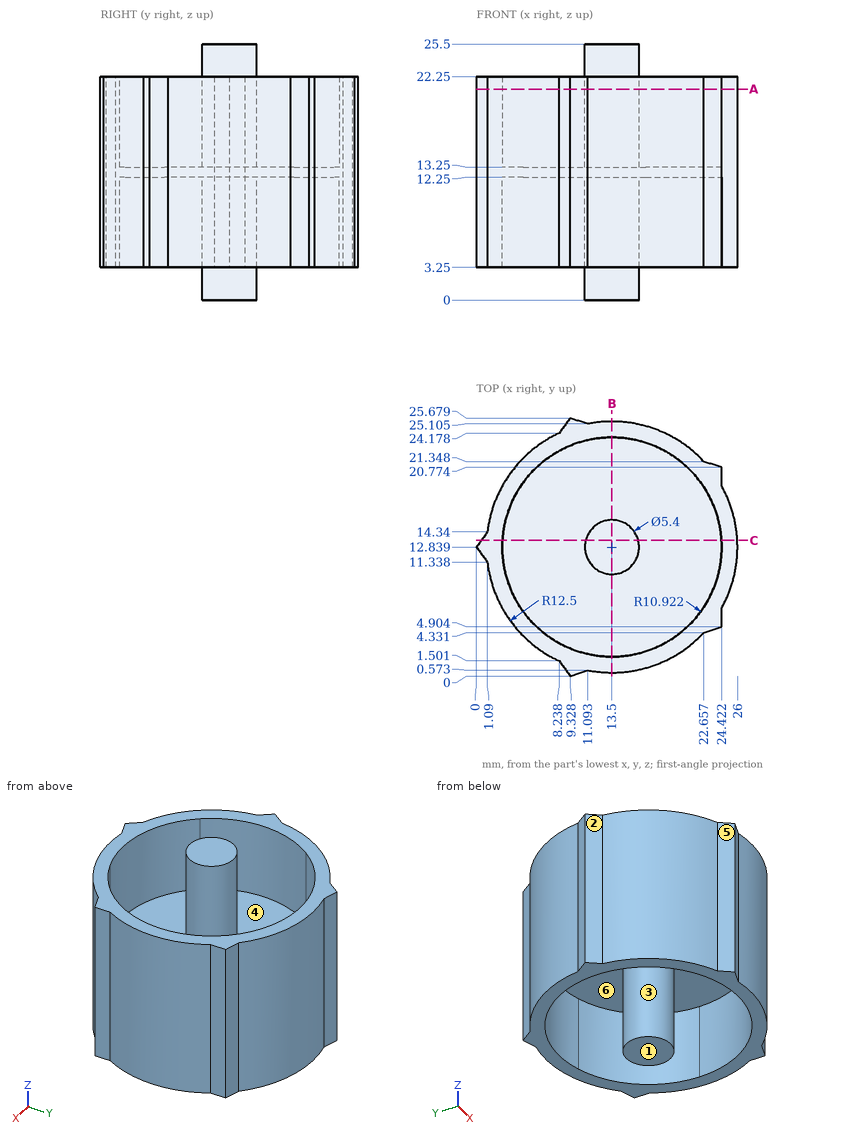
Here's the drawing with two shaded views (mm, measured from the low corner). I have some questions. A direction names the side the tool comes from. Round coordinates to 2 decimals unless told otherwise and drop trailing zeros. Write each loop counter-clockwise with the first axis right and the second up, starting at its lowest first coordinate (ties: lowest second). Pieces come first, ordered by that corner, then holes. Notation, with made-up numbers: M 6,-30.75 L 20,-30.75 A33 cw 20,-2.75 Z; hole C 36.25,43 d3. An arc over 180 degrees is marked long. Use CSV: the item, a comma, the result in double quotes.
(1) We'd pull the mould along X, two halves only. Please class the marked faces 1, 2 and 3: +X half, -X half, draft (parallel to the pull), parting line (faces both ways), or undercut.
Check values:
face 1,"draft"
face 2,"-X half"
face 3,"undercut"
(2) I need wall thicknesses on line 1 along X through (y, z) = (12, 7.75) (1 decimal); line 2 along Z through (x, y) = (8.25, 7.75); line 3 along Y through (x, z) = (22, 21.75) (1 decimal). Which ranges of each line are inside material? Lowest first, please.
Check values:
line 1,"0.6 to 2.6, 10.9 to 16.1, 24.4 to 26"
line 2,"12.25 to 13.25"
line 3,"3.7 to 6, 19.7 to 22"
(3) Imagine slicing it at B-B (x = 13.5). Write out the boundary of the cut face in (y, z).
Check values:
outline,"M 0.34,3.25 L 1.92,3.25 L 1.92,12.25 L 10.14,12.25 L 10.14,0 L 15.54,0 L 15.54,12.25 L 23.76,12.25 L 23.76,3.25 L 25.34,3.25 L 25.34,22.25 L 23.76,22.25 L 23.76,13.25 L 15.54,13.25 L 15.54,25.5 L 10.14,25.5 L 10.14,13.25 L 1.92,13.25 L 1.92,22.25 L 0.34,22.25 Z"
(4) Imagine slicing it at A-A (z = 21). Write out the boundary of the cut face in (x, y) (1 decimal), plus the area to 3 significant figures.
Check values:
outline,"M 0,12.8 L 1.1,11.3 A12.5 ccw 8.2,1.5 L 9.3,0 L 11.1,0.6 A12.5 ccw 22.7,4.3 L 24.4,4.9 L 24.4,6.8 A12.5 ccw 24.4,18.9 L 24.4,20.8 L 22.7,21.3 A12.5 ccw 11.1,25.1 L 9.3,25.7 L 8.2,24.2 A12.5 ccw 1.1,14.3 Z; C 13.5,12.8 d5.4; hole C 13.5,12.8 d21.8"
area,"146 mm^2"
(5) I'm going to push flat-ended pins straight in: pin 1 (0.6 mm diameter, centred on y = 20, z = 12.5, fed in from +X); pin 2 (2 mm diameter, centred on x = 5, y = 5, fed in from -Z); pin 3 (8 mm diameter, centred on x = 22, z = 13.5, fed in from -Y). Where does each tip first touch, or does it pass through?
Check values:
pin 1,"x = 24.42"
pin 2,"z = 3.25"
pin 3,"y = 1.18"
(6) On a 3-axis mill with a long thin cutter (end or side, diameter ignored), from which of +Z, -Z, +X, -X, +Y, -Y can I reach the whole of each face in a straight line? I mean the marked faces 4, 5 and 6. Say none if no direction works.
Check values:
face 4,"+Z"
face 5,"+Z, -Z, -X, -Y"
face 6,"-Z"
(7) Imagine slicing it at C-C (y = 13.5). Write out the boundary of the cut face in (x, z).
Check values:
outline,"M 0.48,3.25 L 2.6,3.25 L 2.6,12.25 L 10.88,12.25 L 10.88,0 L 16.12,0 L 16.12,12.25 L 24.4,12.25 L 24.4,3.25 L 25.98,3.25 L 25.98,22.25 L 24.4,22.25 L 24.4,13.25 L 16.12,13.25 L 16.12,25.5 L 10.88,25.5 L 10.88,13.25 L 2.6,13.25 L 2.6,22.25 L 0.48,22.25 Z"
